Answer from the drawing. Dimensions are ordinates in mm from the lowest x, y and z of the part. A direction names the side the tool comes from. Give positions to 0.01 mm unless a question says otherwise; leave off trailing zeros. Write each loop counter-clockwise with the first axis right and the second up, starting at its lowest first coordinate (ties: lowest second). Pieces come first, ordered by that corner, then holes. Notation, with made-up numbers: (-17, 35) -> (14, 35) arc R12 cw to (14, 45) -> close; hole circle Ø10 at (47.5, 44.5). An arc over 180 degrees is marked (long way). Put each result on its own line as item: value. Start each with the question number.
1) A cutting plane is placed at C-C (z = 2.5). Write down the section's boundary in (x, y) (3 decimals).
2) Flat-ended cylindrical pins translate along their axes: pin 1 Ø4 at (y, z) = (6, 5.5) entering from -X; pin 2 Ø5 at (x, z) = (2.5, 3.5) entering from -Y; pin 3 Ø5 at (x, z) = (16.5, 8) entering from +Y. Find the tip coordinate at first contact, or state that the pin passes through.
3) For a pull along X with two mould halves and no side action, classify the marked faces 4, 5 and 6 as released by +X, released by -X, zero draft, split by the parting line, or undercut.
4) A cutting plane is placed at B-B (x = 10.85). Write down the section's boundary in (y, z) (3 decimals).
5) A cutting plane is placed at A-A (y = 10.85). Write down the section's boundary in (x, z) (3 decimals), then the cut area to 3 significant figures.
6) For the marked faces 1, 2 and 3, determine the directions among +Z, -Z, +X, -X, +Y, -Y from which every point of the face is accessible in a straight line to the end or side of a thin tool.
7) A cutting plane is placed at D-D (x = 16.5). Write down the section's boundary in (y, z), then the cut area to 3 significant figures.
8) Find the intervals of material crossed by line 1 along Y through (x, z) = (10.85, 5.75) (3 decimals); line 2 along Y through (x, z) = (10.85, 6.25) (3 decimals); line 3 along Z through (x, y) = (20, 16.25), in increasing order. Write a range as from..to.
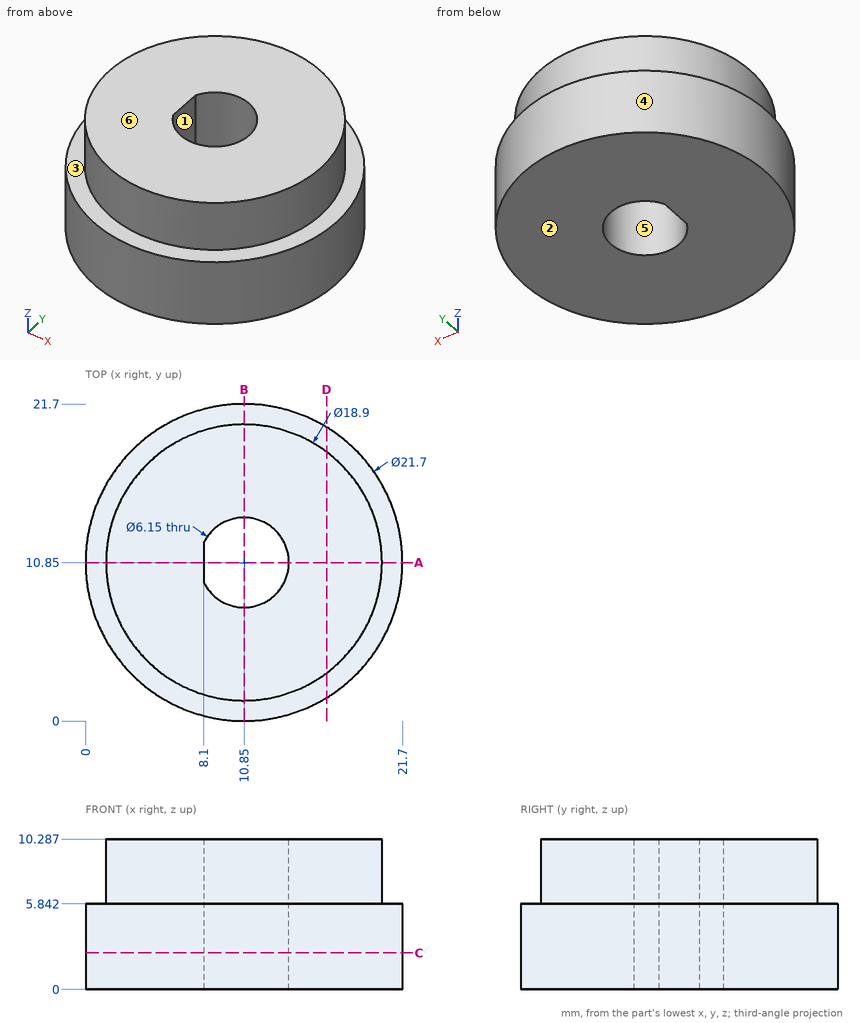
Reply:
1. outline: circle Ø21.7 at (10.85, 10.85); hole (8.1, 9.474) arc R3.075 ccw (long way) to (8.1, 12.226) -> close
2. pin 1: stops at x = 0.38
2. pin 2: stops at y = 1.71
2. pin 3: stops at y = 20.77
3. face 4: split by the parting line
3. face 5: undercut
3. face 6: zero draft
4. outline: (0, 0) -> (7.775, 0) -> (7.775, 10.287) -> (1.4, 10.287) -> (1.4, 5.842) -> (0, 5.842) -> close; (13.925, 0) -> (21.7, 0) -> (21.7, 5.842) -> (20.3, 5.842) -> (20.3, 10.287) -> (13.925, 10.287) -> close
5. outline: (0, 0) -> (8.1, 0) -> (8.1, 10.287) -> (1.4, 10.287) -> (1.4, 5.842) -> (0, 5.842) -> close; (13.925, 0) -> (21.7, 0) -> (21.7, 5.842) -> (20.3, 5.842) -> (20.3, 10.287) -> (13.925, 10.287) -> close
5. area: 151 mm2
6. face 1: +Z, -Z
6. face 2: -Z, +X, -X, +Y, -Y
6. face 3: +Z
7. outline: (1.59, 0) -> (20.11, 0) -> (20.11, 5.84) -> (18.42, 5.84) -> (18.42, 10.29) -> (3.28, 10.29) -> (3.28, 5.84) -> (1.59, 5.84) -> close
7. area: 176 mm2
8. line 1: y = 0..7.775, 13.925..21.7
8. line 2: y = 1.4..7.775, 13.925..20.3
8. line 3: z = 0..5.84
